from build123d import *

# Parameters (mm, degrees)
F1_DEPTH = 50
F0_W     = 25.4
F0_H     = 26.123554
F2_DEPTH = 25.4


with BuildPart() as f1:
    # F0 (on Front) → F1 (new body)
    with BuildSketch(Plane.XZ):
        with BuildLine():
            Line((43.060917, 70.833095), (-71.239083, 70.833095))
            ThreePointArc((-71.239083, 70.833095), (-75.729211, 68.973223), (-77.589083, 64.483095))
            Line((-77.589083, 64.483095), (-77.589083, -19.790707))
            ThreePointArc((-77.589083, -19.790707), (-75.729211, -24.280835), (-71.239083, -26.140707))
            Line((-71.239083, -26.140707), (-26.789083, -26.140707))
            Line((-26.789083, -26.140707), (-1.389083, -26.140707))
            Line((-1.389083, -26.140707), (43.060917, -26.140707))
            ThreePointArc((43.060917, -26.140707), (47.551045, -24.280835), (49.410917, -19.790707))
            Line((49.410917, -19.790707), (49.410917, 64.483095))
            ThreePointArc((49.410917, 64.483095), (47.551045, 68.973223), (43.060917, 70.833095))
        make_face()
    extrude(amount=F1_DEPTH)

    # F0 (on Front) → F2 (join)
    with BuildSketch(Plane.XZ):
        with BuildLine():
            Line((43.060917, 70.833095), (-71.239083, 70.833095))
            ThreePointArc((-71.239083, 70.833095), (-75.729211, 68.973223), (-77.589083, 64.483095))
            Line((-77.589083, 64.483095), (-77.589083, -19.790707))
            ThreePointArc((-77.589083, -19.790707), (-75.729211, -24.280835), (-71.239083, -26.140707))
            Line((-71.239083, -26.140707), (-26.789083, -26.140707))
            Line((-26.789083, -26.140707), (-1.389083, -26.140707))
            Line((-1.389083, -26.140707), (43.060917, -26.140707))
            ThreePointArc((43.060917, -26.140707), (47.551045, -24.280835), (49.410917, -19.790707))
            Line((49.410917, -19.790707), (49.410917, 64.483095))
            ThreePointArc((49.410917, 64.483095), (47.551045, 68.973223), (43.060917, 70.833095))
        make_face()
        with Locations((-14.089083, -39.202484)):
            Rectangle(F0_W, F0_H)
        Polygon((-1.389083, -52.264261), (-26.789083, -52.264261), (-53.967083, -52.264261), (-53.967083, -62.753261), (25.788917, -62.753261), (25.788917, -52.264261), align=None)
    extrude(amount=F2_DEPTH)


solid = f1.part
Source: CAD feature listing. Evaluate the final solid. Frame: model axes, mm. A direction names the side the tool comes from. Give positions to 0.01 mm unless a question says otherwise; leave off trailing zeros. Write each loop counter-clockwise with the first axis right and the second up, starting at its lowest first coordinate (ties: lowest second). Pieces come first, ordered by that corner, then holes. Notation, with made-up numbers: (15.25, 72.5) - (45.25, 72.5) arc R19 ccw to (45.25, 88.5) - close; hole circle Ø11 at (0.5, -17). An arc over 180 degrees is marked (long way). Write item = value, one per line. Start each with the question number.
Q1. Cut plane B-B, the plane y = -17. Return loops of the section in (x, z), then the cut area to 3 significant figures.
Q2. Pin query (flat end, axial travel): pin 1 Ø6 at (x, z) = (24.5, 23) entering from +Y; pin 2 Ø7.5 at (y, z) = (-12, -44.5) entering from -X; pin 3 Ø11 at (x, z) = (-27, -53) entering from -Y; pin 4 Ø5 at (y, z) = (-15.5, -57) entering from +X. Return the tip coordinate at first contact, or that it passes through.
Q3. Cut plane D-D, the plane y = -32.5. Return loops of the section in (x, z).
Q4. Cut plane A-A, the plane x = -34.5. Return loops of the section in (y, z).
Q5. Cut plane C-C, the plane z = -30.5. Return loops of the section in (x, y), then the cut area to 3 significant figures.
Q6. Draft query along Z for faces 1 (the flat face through (-15, -13, -62.753)), 2 (the flat face through (-15, -50, 23)), 3 (the cylindrical face through (-75.7, -24.6, 69)), 4 (the flat face through (12, -13, -52.264)). Return one class per face: +Z half, -Z half, draft (parallel to the pull), parting line (faces both ways), or undercut.
Q7. Reachability of faces 5 (the flat face through (25.789, -13, -58)), 6 (the flat face through (-53.967, -13, -57)), 7 (the flat face through (-15, -25.4, -48)) from +Z, -Z, +X, -X, +Y, -Y: full face, straight path, thin tool, end or side. Return the list, or none.
Q8. Material intervals for probe 1 along Z at (x, y) = (12.5, -19.5); probe 2 along Z at (x, y) = (-47, -36); probe 3 along Y at (x, z) = (-2, -33.5), sorted ascending.
Computed values:
q1.outline = (-77.59, -19.79) arc R6.35 ccw to (-71.24, -26.14) - (-26.79, -26.14) - (-26.79, -52.26) - (-53.97, -52.26) - (-53.97, -62.75) - (25.79, -62.75) - (25.79, -52.26) - (-1.39, -52.26) - (-1.39, -26.14) - (43.06, -26.14) arc R6.35 ccw to (49.41, -19.79) - (49.41, 64.48) arc R6.35 ccw to (43.06, 70.83) - (-71.24, 70.83) arc R6.35 ccw to (-77.59, 64.48) - close
q1.area = 13,800 mm²
q2.pin_1 = 0
q2.pin_2 = -26.79
q2.pin_3 = -25.4
q2.pin_4 = 25.79
q3.outline = (-77.59, -19.79) arc R6.35 ccw to (-71.24, -26.14) - (43.06, -26.14) arc R6.35 ccw to (49.41, -19.79) - (49.41, 64.48) arc R6.35 ccw to (43.06, 70.83) - (-71.24, 70.83) arc R6.35 ccw to (-77.59, 64.48) - close
q4.outline = (-50, -26.14) - (0, -26.14) - (0, 70.83) - (-50, 70.83) - close; (-25.4, -62.75) - (0, -62.75) - (0, -52.26) - (-25.4, -52.26) - close
q5.outline = (-26.79, -25.4) - (-1.39, -25.4) - (-1.39, 0) - (-26.79, 0) - close
q5.area = 645 mm²
q6.face_1 = -Z half
q6.face_2 = draft
q6.face_3 = +Z half
q6.face_4 = undercut
q7.face_5 = -Z, +X, +Y, -Y
q7.face_6 = -Z, -X, +Y, -Y
q7.face_7 = -Z, +X, -X, -Y
q8.probe_1 = -62.75 to -52.26, -26.14 to 70.83
q8.probe_2 = -26.14 to 70.83
q8.probe_3 = -25.4 to 0
